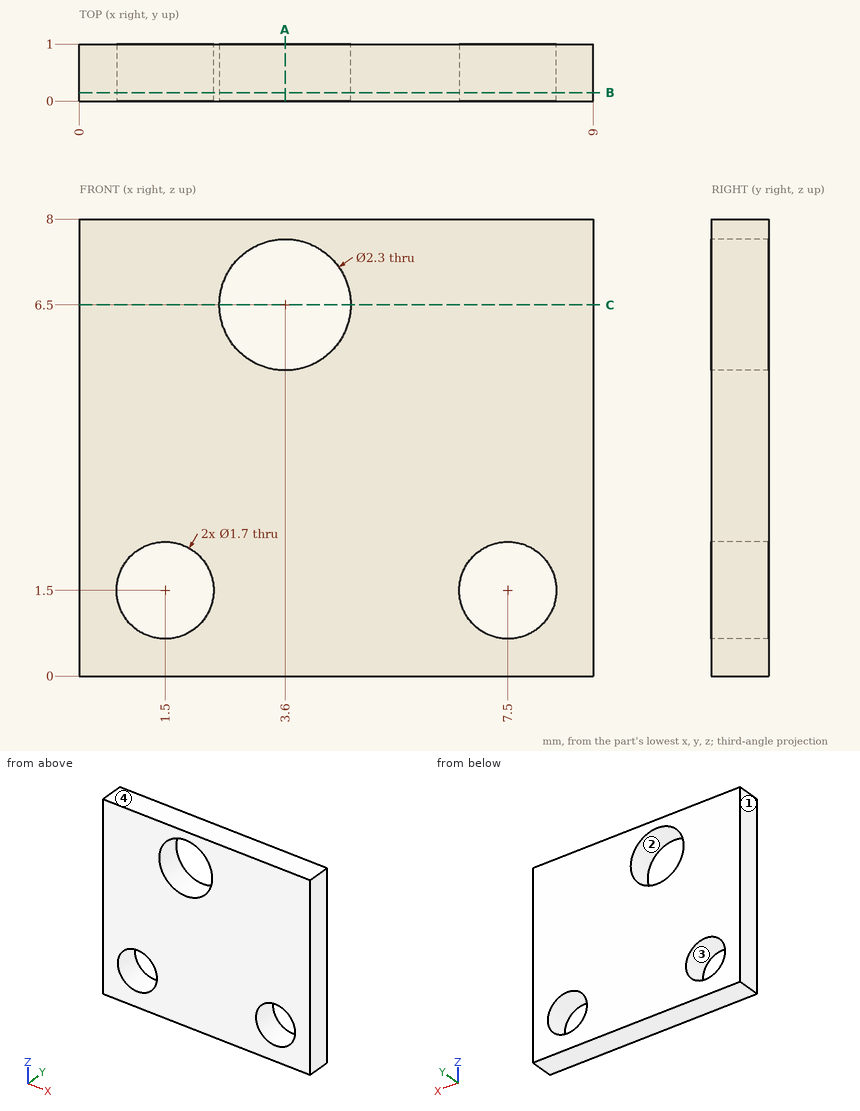
Here's the drawing with two shaded views (mm, measured from the low corner). I have some questions. Round coordinates to 2 decimals unless told otherwise and drop trailing zeros. Loops run counter-clockwise (first coordinate to the right, second up) from the corner with the lowest first, then second, coordinate; pieces in that order, holes last.
Item 1: If we mould it in two halves opening along X, with no side actions, what happens to the marked faces 1, 2, 3 and 4? For each: +X half, -X half, draft (parallel to the pull), parting line (faces both ways), or undercut.
Item 2: Suppose I cut it at B-B, the plane y = 0.15. Write out the boundary of the cut face in (x, z), then the cut area to 3 significant figures.
Item 3: Suppose I cut it at C-C, the plane z = 6.5. Write out the boundary of the cut face in (x, y).
Item 4: Please list where these lines run through material, in increasing order: L1, parallel to X at y = 0.6, z = 1.5; L2, parallel to X at y = 0.45, z = 6.5; L3, parallel to Z at x = 3.6, y = 0.4.
Item 5: Will this pin go through, and if not, where does the flat tip stop? pin 1 Ø1.8 at (x, z) = (3.6, 6.5) entering from -Y.
Item 6: Suppose I cut it at A-A, the plane x = 3.6. Write out the boundary of the cut face in (y, z).
Reported:
1. face 1: -X half
1. face 2: undercut
1. face 3: undercut
1. face 4: draft
2. outline: (0, 0) - (9, 0) - (9, 8) - (0, 8) - close; hole circle Ø1.7 at (1.5, 1.5); hole circle Ø2.3 at (3.6, 6.5); hole circle Ø1.7 at (7.5, 1.5)
2. area: 63.3 mm2
3. outline: (0, 0) - (2.45, 0) - (2.45, 1) - (0, 1) - close; (4.75, 0) - (9, 0) - (9, 1) - (4.75, 1) - close
4. L1: x = 0 to 0.65, 2.35 to 6.65, 8.35 to 9
4. L2: x = 0 to 2.45, 4.75 to 9
4. L3: z = 0 to 5.35, 7.65 to 8
5. pin 1: passes through
6. outline: (0, 0) - (1, 0) - (1, 5.35) - (0, 5.35) - close; (0, 7.65) - (1, 7.65) - (1, 8) - (0, 8) - close
